Geometry: final body of the model. Coordinates: model frame, mm. Give positions to 0.01 mm unless a question says otherwise; leave off trailing zeros.
from build123d import *

# Parameters (mm, degrees)
SKETCH1_W           = 239.388843642
SKETCH1_H           = 75.842411424
BOSS_EXTRUDE1_DEPTH = 1.5875
CUT_EXTRUDE1_REACH  = 127.568
SKETCH2_R           = 4.1275
SKETCH2_R_2         = 4.572
SKETCH2_R_3         = 4.0513
SKETCH2_W           = 14.8082
SKETCH2_H           = 7.0104
SKETCH2_W_2         = 15.9004
SKETCH2_H_2         = 7.8232
SKETCH2_W_3         = 15.24
SKETCH2_H_3         = 12.2174
SKETCH2_H_4         = 6.8072


with BuildPart() as part:
    # Sketch1 → Boss-Extrude1 (new body)
    with BuildSketch(Plane(origin=(0, 0, 0), x_dir=(1, 0, 0), z_dir=(0, 1, 0))):
        Rectangle(SKETCH1_W, SKETCH1_H)
    extrude(amount=-BOSS_EXTRUDE1_DEPTH)

    # Sketch2 → Cut-Extrude1 (cut, up to next)
    with BuildSketch(Plane(origin=(0, 0, 0), x_dir=(1, 0, 0), z_dir=(0, 1, 0)), mode=Mode.PRIVATE) as cut_extrude1_sk1:
        with Locations(Location((-75.244421821, -22.046205712, 0), (0, 0, 270))):
            Circle(SKETCH2_R)
    cut_extrude1_tool1 = extrude(cut_extrude1_sk1.sketch, amount=-CUT_EXTRUDE1_REACH, mode=Mode.PRIVATE) & part.part
    # Sketch2 → Cut-Extrude1 (cut, up to next)
    with BuildSketch(Plane(origin=(0, 0, 0), x_dir=(1, 0, 0), z_dir=(0, 1, 0)), mode=Mode.PRIVATE) as cut_extrude1_sk2:
        with Locations(Location((49.507678179, -25.713445712, 0), (0, 0, 270))):
            Circle(SKETCH2_R_2)
    cut_extrude1_tool2 = extrude(cut_extrude1_sk2.sketch, amount=-CUT_EXTRUDE1_REACH, mode=Mode.PRIVATE) & part.part
    # Sketch2 → Cut-Extrude1 (cut, up to next)
    with BuildSketch(Plane(origin=(0, 0, 0), x_dir=(1, 0, 0), z_dir=(0, 1, 0)), mode=Mode.PRIVATE) as cut_extrude1_sk3:
        with Locations(Location((-75.244421821, -6.171205712, 0), (0, 0, 270))):
            Circle(SKETCH2_R_3)
    cut_extrude1_tool3 = extrude(cut_extrude1_sk3.sketch, amount=-CUT_EXTRUDE1_REACH, mode=Mode.PRIVATE) & part.part
    # Sketch2 → Cut-Extrude1 (cut, up to next)
    with BuildSketch(Plane(origin=(0, 0, 0), x_dir=(1, 0, 0), z_dir=(0, 1, 0)), mode=Mode.PRIVATE) as cut_extrude1_sk4:
        with Locations(Location((49.507678179, -3.869445712, 0), (0, 0, 270))):
            Circle(SKETCH2_R_2)
    cut_extrude1_tool4 = extrude(cut_extrude1_sk4.sketch, amount=-CUT_EXTRUDE1_REACH, mode=Mode.PRIVATE) & part.part
    # Sketch2 → Cut-Extrude1 (cut, up to next)
    with BuildSketch(Plane(origin=(0, 0, 0), x_dir=(1, 0, 0), z_dir=(0, 1, 0)), mode=Mode.PRIVATE) as cut_extrude1_sk5:
        with Locations(Location((61.572678179, -3.869445712, 0), (0, 0, 270))):
            Circle(SKETCH2_R_2)
    cut_extrude1_tool5 = extrude(cut_extrude1_sk5.sketch, amount=-CUT_EXTRUDE1_REACH, mode=Mode.PRIVATE) & part.part
    # Sketch2 → Cut-Extrude1 (cut, up to next)
    with BuildSketch(Plane(origin=(0, 0, 0), x_dir=(1, 0, 0), z_dir=(0, 1, 0)), mode=Mode.PRIVATE) as cut_extrude1_sk6:
        with Locations(Location((49.507678179, -14.893045712, 0), (0, 0, 270))):
            Circle(SKETCH2_R_2)
    cut_extrude1_tool6 = extrude(cut_extrude1_sk6.sketch, amount=-CUT_EXTRUDE1_REACH, mode=Mode.PRIVATE) & part.part
    # Sketch2 → Cut-Extrude1 (cut, up to next)
    with BuildSketch(Plane(origin=(0, 0, 0), x_dir=(1, 0, 0), z_dir=(0, 1, 0)), mode=Mode.PRIVATE) as cut_extrude1_sk7:
        with Locations(Location((61.572678179, -14.893045712, 0), (0, 0, 270))):
            Circle(SKETCH2_R_2)
    cut_extrude1_tool7 = extrude(cut_extrude1_sk7.sketch, amount=-CUT_EXTRUDE1_REACH, mode=Mode.PRIVATE) & part.part
    # Sketch2 → Cut-Extrude1 (cut, up to next)
    with BuildSketch(Plane(origin=(0, 0, 0), x_dir=(1, 0, 0), z_dir=(0, 1, 0)), mode=Mode.PRIVATE) as cut_extrude1_sk8:
        with Locations(Location((61.572678179, -25.713445712, 0), (0, 0, 270))):
            Circle(SKETCH2_R_2)
    cut_extrude1_tool8 = extrude(cut_extrude1_sk8.sketch, amount=-CUT_EXTRUDE1_REACH, mode=Mode.PRIVATE) & part.part
    # Sketch2 → Cut-Extrude1 (cut, up to next)
    with BuildSketch(Plane(origin=(0, 0, 0), x_dir=(1, 0, 0), z_dir=(0, 1, 0)), mode=Mode.PRIVATE) as cut_extrude1_sk9:
        Polygon((-47.558421821, -25.977996251), (-31.683421821, -25.977996251), (-31.683421821, -30.60665864), (-34.032921821, -32.251796251), (-45.208921821, -32.251796251), (-47.558421821, -30.60665864), align=None)
    cut_extrude1_tool9 = extrude(cut_extrude1_sk9.sketch, amount=-CUT_EXTRUDE1_REACH, mode=Mode.PRIVATE) & part.part
    # Sketch2 → Cut-Extrude1 (cut, up to next)
    with BuildSketch(Plane(origin=(0, 0, 0), x_dir=(1, 0, 0), z_dir=(0, 1, 0)), mode=Mode.PRIVATE) as cut_extrude1_sk10:
        with BuildLine():
            Line((-52.955921821, -14.154296251), (-52.955921821, -15.817996251))
            Line((-52.955921821, -15.817996251), (-26.285921821, -15.817996251))
            Line((-26.285921821, -15.817996251), (-26.285921821, -14.154296251))
            Line((-26.285921821, -14.154296251), (-23.479221821, -14.154296251))
            ThreePointArc((-23.479221821, -14.154296251), (-20.126421821, -10.801496251), (-23.479221821, -7.448696251))
            Line((-23.479221821, -7.448696251), (-26.285921821, -7.448696251))
            Line((-26.285921821, -7.448696251), (-26.285921821, -5.784996251))
            Line((-26.285921821, -5.784996251), (-52.955921821, -5.784996251))
            Line((-52.955921821, -5.784996251), (-52.955921821, -7.448696251))
            Line((-52.955921821, -7.448696251), (-55.762621821, -7.448696251))
            ThreePointArc((-55.762621821, -7.448696251), (-59.115421821, -10.801496251), (-55.762621821, -14.154296251))
            Line((-55.762621821, -14.154296251), (-52.955921821, -14.154296251))
        make_face()
    cut_extrude1_tool10 = extrude(cut_extrude1_sk10.sketch, amount=-CUT_EXTRUDE1_REACH, mode=Mode.PRIVATE) & part.part
    # Sketch2 → Cut-Extrude1 (cut, up to next)
    with BuildSketch(Plane(origin=(0, 0, 0), x_dir=(1, 0, 0), z_dir=(0, 1, 0)), mode=Mode.PRIVATE) as cut_extrude1_sk11:
        with Locations((3.401875226, -11.222745712)):
            Rectangle(SKETCH2_W, SKETCH2_H)
    cut_extrude1_tool11 = extrude(cut_extrude1_sk11.sketch, amount=-CUT_EXTRUDE1_REACH, mode=Mode.PRIVATE) & part.part
    # Sketch2 → Cut-Extrude1 (cut, up to next)
    with BuildSketch(Plane(origin=(0, 0, 0), x_dir=(1, 0, 0), z_dir=(0, 1, 0)), mode=Mode.PRIVATE) as cut_extrude1_sk12:
        with Locations((3.401875226, -19.934945712)):
            Rectangle(SKETCH2_W, SKETCH2_H)
    cut_extrude1_tool12 = extrude(cut_extrude1_sk12.sketch, amount=-CUT_EXTRUDE1_REACH, mode=Mode.PRIVATE) & part.part
    # Sketch2 → Cut-Extrude1 (cut, up to next)
    with BuildSketch(Plane(origin=(0, 0, 0), x_dir=(1, 0, 0), z_dir=(0, 1, 0)), mode=Mode.PRIVATE) as cut_extrude1_sk13:
        with Locations((3.401875226, -29.002745712)):
            Rectangle(SKETCH2_W_2, SKETCH2_H_2)
    cut_extrude1_tool13 = extrude(cut_extrude1_sk13.sketch, amount=-CUT_EXTRUDE1_REACH, mode=Mode.PRIVATE) & part.part
    # Sketch2 → Cut-Extrude1 (cut, up to next)
    with BuildSketch(Plane(origin=(0, 0, 0), x_dir=(1, 0, 0), z_dir=(0, 1, 0)), mode=Mode.PRIVATE) as cut_extrude1_sk14:
        with Locations((30.610078179, -8.596905712)):
            Rectangle(SKETCH2_W_3, SKETCH2_H_3)
    cut_extrude1_tool14 = extrude(cut_extrude1_sk14.sketch, amount=-CUT_EXTRUDE1_REACH, mode=Mode.PRIVATE) & part.part
    # Sketch2 → Cut-Extrude1 (cut, up to next)
    with BuildSketch(Plane(origin=(0, 0, 0), x_dir=(1, 0, 0), z_dir=(0, 1, 0)), mode=Mode.PRIVATE) as cut_extrude1_sk15:
        with Locations((30.610078179, -19.811005712)):
            Rectangle(SKETCH2_W_3, SKETCH2_H_4)
    cut_extrude1_tool15 = extrude(cut_extrude1_sk15.sketch, amount=-CUT_EXTRUDE1_REACH, mode=Mode.PRIVATE) & part.part
    # Sketch2 → Cut-Extrude1 (cut, up to next)
    with BuildSketch(Plane(origin=(0, 0, 0), x_dir=(1, 0, 0), z_dir=(0, 1, 0)), mode=Mode.PRIVATE) as cut_extrude1_sk16:
        with Locations((30.610078179, -28.320005712)):
            Rectangle(SKETCH2_W_3, SKETCH2_H_4)
    cut_extrude1_tool16 = extrude(cut_extrude1_sk16.sketch, amount=-CUT_EXTRUDE1_REACH, mode=Mode.PRIVATE) & part.part
    add(cut_extrude1_tool1.solids().sort_by_distance((-75.244422, 0, 22.046206))[0], mode=Mode.SUBTRACT)
    add(cut_extrude1_tool2.solids().sort_by_distance((49.507678, 0, 25.713446))[0], mode=Mode.SUBTRACT)
    add(cut_extrude1_tool3.solids().sort_by_distance((-75.244422, 0, 6.171206))[0], mode=Mode.SUBTRACT)
    add(cut_extrude1_tool4.solids().sort_by_distance((49.507678, 0, 3.869446))[0], mode=Mode.SUBTRACT)
    add(cut_extrude1_tool5.solids().sort_by_distance((61.572678, 0, 3.869446))[0], mode=Mode.SUBTRACT)
    add(cut_extrude1_tool6.solids().sort_by_distance((49.507678, 0, 14.893046))[0], mode=Mode.SUBTRACT)
    add(cut_extrude1_tool7.solids().sort_by_distance((61.572678, 0, 14.893046))[0], mode=Mode.SUBTRACT)
    add(cut_extrude1_tool8.solids().sort_by_distance((61.572678, 0, 25.713446))[0], mode=Mode.SUBTRACT)
    add(cut_extrude1_tool9.solids().sort_by_distance((-39.620922, 0, 29.010382))[0], mode=Mode.SUBTRACT)
    add(cut_extrude1_tool10.solids().sort_by_distance((-39.620922, 0, 10.801496))[0], mode=Mode.SUBTRACT)
    add(cut_extrude1_tool11.solids().sort_by_distance((3.401875, 0, 11.222746))[0], mode=Mode.SUBTRACT)
    add(cut_extrude1_tool12.solids().sort_by_distance((3.401875, 0, 19.934946))[0], mode=Mode.SUBTRACT)
    add(cut_extrude1_tool13.solids().sort_by_distance((3.401875, 0, 29.002746))[0], mode=Mode.SUBTRACT)
    add(cut_extrude1_tool14.solids().sort_by_distance((30.610078, 0, 8.596906))[0], mode=Mode.SUBTRACT)
    add(cut_extrude1_tool15.solids().sort_by_distance((30.610078, 0, 19.811006))[0], mode=Mode.SUBTRACT)
    add(cut_extrude1_tool16.solids().sort_by_distance((30.610078, 0, 28.320006))[0], mode=Mode.SUBTRACT)


solid = part.part
Q1. Pull-direction query (X, two-part tool) for faces 1 (the flat face through (-2, -1.588, -1)), 2 (the cylindrical face through (-71.15, -0.78, 21.51)), 3 (the cylindrical face through (50.881, -0.783, 30.074)); classes: released by +X, released by -X, zero draft, split by the parting line, or undercut.
Filled sheet:
face 1: zero draft
face 2: undercut
face 3: undercut
Q2. Pin query (flat end, axial travel): P1, Ø10.5, axis at x = -75.24, z = 22.05, coming from the +Y side. Return the tip coordinate at first contact, or that it passes through.
Filled sheet:
P1: stops at y = 0
Q3. Ray query, line 1 along Z through (x, y) = (30.5, -0.35); line 2 along Z through (x, y) = (-75, -0.5); line 3 along X through (y, z) = (-1, 5). Return the intervals inside material, ascending.
Filled sheet:
line 1: z = -37.92 to 2.49, 14.71 to 16.41, 23.21 to 24.92, 31.72 to 37.92
line 2: z = -37.92 to 2.13, 10.22 to 17.93, 26.17 to 37.92
line 3: x = -119.69 to -79.12, -71.37 to 22.99, 38.23 to 45.08, 53.94 to 57.14, 66 to 119.69
Q4. Section A-A on y = -0.45. Count the separate pieces of the cut face and the enclosed holes in it, plus the area to 3 significant figures.
Filled sheet:
separate pieces: 1
enclosed holes: 16
area: 16,500 mm2
